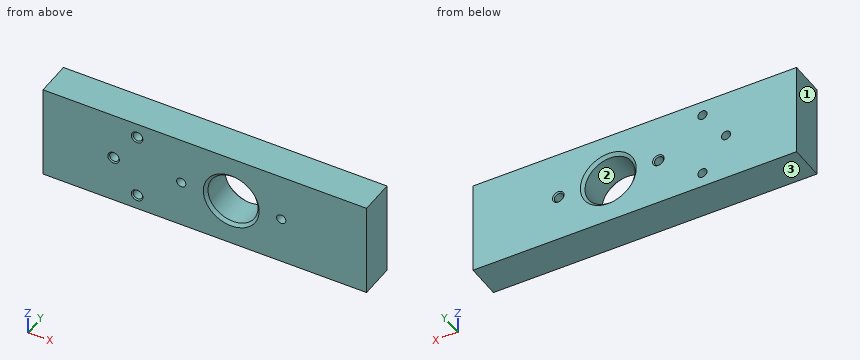
Autodesk Inventor part; units mm, degrees
ref_plane "YZ Plane" through (0, 0, 0) normal (1, 0, 0) x (0, 1, 0)
ref_plane "XZ Plane" through (0, 0, 0) normal (0, 1, 0) x (-1, 0, 0)
ref_plane "XY Plane" through (0, 0, 0) normal (0, 0, 1) x (1, 0, 0)
sketch "Sketch1" plane through (0, 0, 0) normal (0, 1, 0) x (-1, 0, 0)
  line L0 (-27.5, 8) -> (27.5, 8)
  line L1 (27.5, 8) -> (27.5, -8)
  line L2 (27.5, -8) -> (-27.5, -8)
  line L3 (-27.5, -8) -> (-27.5, 8)
  line L4 (-27.5, 8) -> (27.5, -8) construction
  line L5 (27.5, 8) -> (-27.5, -8) construction
  point P0 (0, 0)
  dimension "d0" = 55
  dimension "d1" = 16
extrude "Extrusion1" add sketch "Sketch1" along normal blind 6
sketch "Sketch2" plane through (0, 6, 0) normal (0, 1, 0) x (1, 0, 0)
  line L0 (27.5, 8) -> (-27.5, 8) construction
  line L1 (-27.5, 8) -> (-27.5, -8) construction
  line L2 (-27.5, -8) -> (27.5, -8) construction
  line L3 (27.5, -8) -> (27.5, 8) construction
  point P0 (0, 0)
  point P1 (4.5, 0)
  dimension "d4" = 23
hole "Hole1" at (4.5, 6, 0) direction (0, -1, 0) diameter 8.5 end through all
chamfer "Chamfer1" distance 0.5 angle 45 2 edges at (4.5, 0, -4.25) (4.5, 6, -4.25)
sketch "Sketch3" plane through (0, 6, 0) normal (0, 1, 0) x (1, 0, 0)
  circle A0 centre (-15.5, 0) radius 1.4 construction
  line L0 (-18.5, 8) -> (-4.5, 8) construction
  line L1 (-4.5, 8) -> (-4.5, -8) construction
  line L2 (-4.5, -8) -> (-18.5, -8) construction
  line L3 (-18.5, 8) -> (-18.5, -8)
  circle A1 centre (-11.5, 5.5) radius 1.4
  circle A2 centre (-11.5, -5.5) radius 1.4
  point P0 (0, 0)
  point P1 (-15.5, 0)
hole "Hole2" at (-15.5, 6, 0) at (-11.5, 6, -5.5) at (-11.5, 6, 5.5) direction (0, -1, 0) diameter 1.567 end through all
chamfer "Chamfer2" distance 0.2 angle 45 3 edges at (-11.5, 0, -6.2835) (-15.5, 0, -0.7835) (-11.5, 0, 4.7165)
sketch "Sketch4" plane through (0, 6, 0) normal (0, 1, 0) x (1, 0, 0)
  circle A0 centre (-4, 0) radius 2.2 construction
  circle A1 centre (13, 0) radius 2.2 construction
  point P0 (0, 0)
hole "Hole3" at (-4, 6, 0) at (13, 6, 0) direction (0, -1, 0) diameter 1.567 end through all
chamfer "Chamfer3" distance 0.2 angle 45 2 edges at (13, 6, -0.7835) (-4, 6, -0.7835)
properties part number "KN-00-02-11" material "X5CrNi18-10"
For this review, take the finished solid that the model builds, in its own axes (mm). Face numbers are marked on the shaded views. Round coordinates to 2 decimals unless told otherwise and drop trailing zeros. Loops run counter-clockwise (first coordinate to the right, second up) from the corner with the lowest first, then second, coordinate; pieces in that order, holes last.
(1) Mouldability with a two-part tool opening along X and no side actions: class the marked faces 1, 2 and 3 as released by +X, released by -X, zero draft, split by the parting line, or undercut.
Returned:
face 1: released by -X
face 2: undercut
face 3: zero draft
(2) Wall thickness on line 1 along X through (y, z) = (4.25, 0); line 2 along Z through (x, y) = (4.5, 3.7); line 3 along X through (y, z) = (3.7, -5.5): over which ranges is each line inside the solid? List them lowest first.
Returned:
line 1: x = -27.5 to -16.28, -14.72 to -4.78, -3.22 to 0.25, 8.75 to 12.22, 13.78 to 27.5
line 2: z = -8 to -4.25, 4.25 to 8
line 3: x = -27.5 to -12.28, -10.72 to 27.5
(3) We need section D-D (z = 5.5). Give the boundary of the cut face in (x, y), plus the area to 3 significant figures.
Returned:
outline: (-27.5, 0) - (-12.48, 0) - (-12.28, 0.2) - (-12.28, 6) - (-27.5, 6) - close; (-10.72, 0.2) - (-10.52, 0) - (27.5, 0) - (27.5, 6) - (-10.72, 6) - close
area: 321 mm2
(4) We need section A-A (z = 0). State how many separate pieces and enclosed holes the cut face has, plus the area to 3 significant figures.
Returned:
separate pieces: 5
enclosed holes: 0
area: 250 mm2
(5) We need section B-B (x = 13). Give the boundary of the cut face in (y, z).
Returned:
outline: (0, -8) - (6, -8) - (6, -0.98) - (5.8, -0.78) - (0, -0.78) - close; (0, 0.78) - (5.8, 0.78) - (6, 0.98) - (6, 8) - (0, 8) - close
(6) We need section C-C (y = 1.3). Give the boundary of the cut face in (x, z).
Returned:
outline: (-27.5, -8) - (27.5, -8) - (27.5, 8) - (-27.5, 8) - close; hole circle Ø1.57 at (-15.5, 0); hole circle Ø1.57 at (-11.5, -5.5); hole circle Ø1.57 at (-11.5, 5.5); hole circle Ø1.57 at (-4, 0); hole circle Ø8.5 at (4.5, 0); hole circle Ø1.57 at (13, 0)
(7) Clearance check with flat-ended pins moving along their axes: P1, Ø1.3, axis at x = -11.5, z = -5.5, coming from the -Y side; P2, Ø1.8, axis at x = -4, z = 0, coming from the +Y side. State where each tip first meets the part, or that it passes through.
Returned:
P1: passes through
P2: stops at y = 5.92
